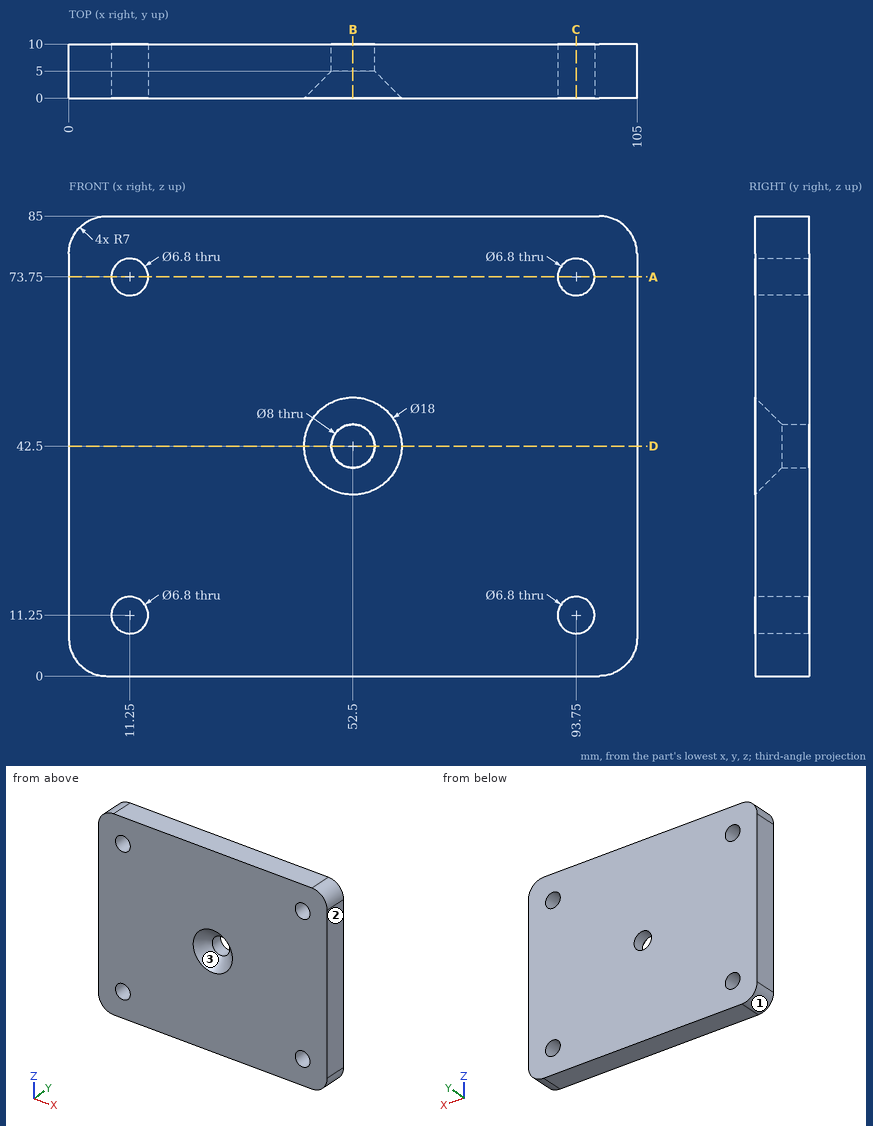
Print and shaded views of the part. All mm, measured from the part's lowest x, y and z. Coordinates: 2 decimals unless noted, no trailing zeros. Loops run counter-clockwise (first coordinate to the right, second up) from the corner with the lowest first, then second, coordinate; pieces in that order, holes last. Notation, with made-up numbers: (36, -13.5) - (51, -13.5) arc R25 ccw to (51, 20.5) - close; hole circle Ø3 at (6.25, 65.25). An arc over 180 degrees is marked (long way). Use one line per item in the form item = value. Start each with the question number.
1) Two-plate mould, pull along Z, no slides. Class the marked faces 1, 2 and 3: +Z half, -Z half, draft (parallel to the pull), parting line (faces both ways), or undercut.
2) Band-saw the part on C-C (x = 93.75). Give the cut face in (y, z), and give its area (3 significant figures).
3) Band-saw the part on B-B (x = 52.5). Give the cut face in (y, z).
4) Drill centre lines: L1, parallel to Z at x = 93.75, y = 4; L2, parallel to X at y = 4.5, z = 11.25; L3, parallel to Z at x = 91, y = 3.5. Where is each one in solid material? Low to high. Write a range as from..to.
5) Band-saw the part on A-A (z = 73.75). Give the cut face in (x, y).
6) Band-saw the part on D-D (z = 42.5). Give the cut face in (x, y).
7) Flat gauge pin, fed straight in: pin 1 (4 mm diameter, centred on x = 93.75, z = 73.75, fed in from -Y). Where does the tip first touch, or does it go through?
Check values:
q1.face_1 = -Z half
q1.face_2 = draft
q1.face_3 = undercut
q2.outline = (0, 0) - (10, 0) - (10, 7.85) - (0, 7.85) - close; (0, 14.65) - (10, 14.65) - (10, 70.35) - (0, 70.35) - close; (0, 77.15) - (10, 77.15) - (10, 85) - (0, 85) - close
q2.area = 714 mm2
q3.outline = (0, 0) - (10, 0) - (10, 38.5) - (5, 38.5) - (0, 33.5) - close; (0, 51.5) - (5, 46.5) - (10, 46.5) - (10, 85) - (0, 85) - close
q4.L1 = 0..7.85, 14.65..70.35, 77.15..85
q4.L2 = 0..7.85, 14.65..90.35, 97.15..105
q4.L3 = 0..9.25, 13.25..71.75, 75.75..85
q5.outline = (0, 0) - (7.85, 0) - (7.85, 10) - (0, 10) - close; (14.65, 0) - (90.35, 0) - (90.35, 10) - (14.65, 10) - close; (97.15, 0) - (105, 0) - (105, 10) - (97.15, 10) - close
q6.outline = (0, 0) - (43.5, 0) - (48.5, 5) - (48.5, 10) - (0, 10) - close; (56.5, 5) - (61.5, 0) - (105, 0) - (105, 10) - (56.5, 10) - close
q7.pin_1 = through
